Check sheet for the modelled part. Datum: model origin and axes. Units: mm. Face numbers are marked on the shaded views. A direction names the side the tool comes from. Give positions to 0.01 mm unless a question says otherwise; leave off trailing zeros. Order: outer loops, then holes, each group sorted by start corner. A loop starts at its lowest first (then second) coordinate and runs counter-clockwise, first axis right, second up. Notation, with made-up numbers: (-21, 57) -> (28, 57) arc R34 cw to (28, 94) -> close; hole circle Ø7 at (50.25, 44.25). An arc over 180 degrees is marked (long way). Answer in a Markdown table with one row per item. Add a question column.
(1) Thickness scan on L1, parallel to X at y = -0.5, z = -4.5 (3 decimals); L2, parallel to Y at x = -24.5, z = 0.75 (3 decimals); L3, parallel to Y at x = 0, z = 4.1 (3 decimals). Record the ranges inside material, lowest first. Write a range as [from, to].
(2) Set-up check for the marked faces 1 and 2: record each of +Z, -Z, +X, -X, +Y, -Y from which the full face is reachable in a straight line by a thin tool's end or side.
(3) Cross-section at A-A (x = 0). Record the cut outline in (y, z) (3 decimals).
(4) Cross-section at D-D (x = -21.5). Record the cut outline in (y, z) (3 decimals), then the cut area to 3 significant figures.
(5) Release check for a two-part mould opening along Y. For the marked faces 3, 4 and 5 record: released by +Y, released by -Y, zero draft, split by the parting line, or undercut.
(6) Cross-section at C-C (y = 2.25). Record the cut outline in (x, z) (3 decimals).
(7) Cross-section at B-B (z = -3.5). Record the cut outline in (x, y) (3 decimals), then the cut area to 3 significant figures.
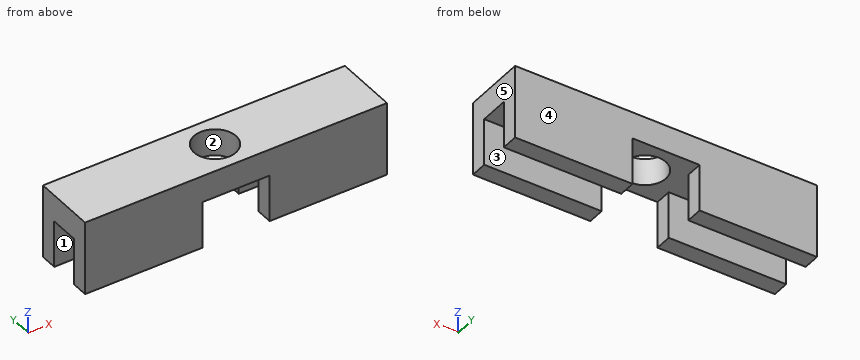
```python
from build123d import *

# Parameters (mm, degrees)
F0_W     = 57.15
F0_H     = 13.97
F1_DEPTH = 3.175
F2_W     = 57.15
F2_H     = 5.08
F3_DEPTH = 2.778125
F5_R     = 3.96875
F6_DEPTH = 13.971
F7_W     = 12.7
F7_H     = 11.90625
F8_DEPTH = 8.89


with BuildPart() as f1:
    # F0 (on Front) → F1 (new body)
    with BuildSketch(Plane.XZ):
        Rectangle(F0_W, F0_H)
    extrude(amount=F1_DEPTH)

    # F2 (on face) → F3 (join)
    with BuildSketch(Plane(origin=(0, 0, 0), x_dir=(-1, 0, 0), z_dir=(0, 1, 0))):
        with Locations((0, 4.445)):
            Rectangle(F2_W, F2_H)
    extrude(amount=F3_DEPTH)

    # F4: F1 across face


with BuildPart() as f1_1:
    add(f1.part)
    add(f1.part.mirror(Plane(origin=(0, 2.778125, 4.445), x_dir=(-1, 0, 0), z_dir=(0, 1, 0))))

    # F5 (on face) → F6 (cut, through all)
    with BuildSketch(Plane.XY.offset(6.985)):
        with Locations((0, 2.778125)):
            Circle(F5_R)
    extrude(amount=-F6_DEPTH, mode=Mode.SUBTRACT)

    # F7 (on face) → F8 (cut)
    with BuildSketch(Plane(origin=(0, 0, -6.985), x_dir=(1, 0, 0), z_dir=(0, 0, -1))):
        with Locations((0, -2.778125)):
            Rectangle(F7_W, F7_H)
    extrude(amount=-F8_DEPTH, mode=Mode.SUBTRACT)


solid = f1_1.part
```
Answer below:
| question | item | result |
|---|---|---|
| 1 | L1 | x = [-28.575, -6.35], [6.35, 28.575] |
| 1 | L2 | y = [-3.175, 0], [5.556, 8.731] |
| 1 | L3 | y = [-3.175, -1.191], [6.747, 8.731] |
| 2 | face 1 | -Z, +X, -X |
| 2 | face 2 | +Z, -Z |
| 3 | outline | (-3.175, 1.905) -> (-1.191, 1.905) -> (-1.191, 6.985) -> (-3.175, 6.985) -> close; (6.747, 1.905) -> (8.731, 1.905) -> (8.731, 6.985) -> (6.747, 6.985) -> close |
| 4 | outline | (-3.175, -6.985) -> (0, -6.985) -> (0, 1.905) -> (5.556, 1.905) -> (5.556, -6.985) -> (8.731, -6.985) -> (8.731, 6.985) -> (-3.175, 6.985) -> close |
| 4 | area | 117 mm² |
| 5 | face 3 | undercut |
| 5 | face 4 | released by +Y |
| 5 | face 5 | zero draft |
| 6 | outline | (-28.575, 1.905) -> (-3.933, 1.905) -> (-3.933, 6.985) -> (-28.575, 6.985) -> close; (3.933, 1.905) -> (28.575, 1.905) -> (28.575, 6.985) -> (3.933, 6.985) -> close |
| 7 | outline | (-28.575, -3.175) -> (-6.35, -3.175) -> (-6.35, 0) -> (-28.575, 0) -> close; (-28.575, 5.556) -> (-6.35, 5.556) -> (-6.35, 8.731) -> (-28.575, 8.731) -> close; (6.35, -3.175) -> (28.575, -3.175) -> (28.575, 0) -> (6.35, 0) -> close; (6.35, 5.556) -> (28.575, 5.556) -> (28.575, 8.731) -> (6.35, 8.731) -> close |
| 7 | area | 282 mm² |
